from build123d import *

# Parameters (mm, degrees)
SKETCH1_W                    = 406.4
SKETCH1_H                    = 44.196
BASE_FLANGE1_DEPTH           = 1.88
EDGE_FLANGE1_STRIP_W         = 8.9932
EDGE_FLANGE1_STRIP_H         = 1.88
EDGE_FLANGE1_STRIP_CUT_DEPTH = 44.196
EDGE_FLANGE1_DEPTH           = 44.196
CUT_EXTRUDE1_REACH           = 411.347
FILLET1_R                    = 5


# Sheet-metal steps are written as plain solids
with BuildPart() as part:
    # Sketch1 → Base-Flange1 (new body)
    with BuildSketch(Plane.XY):
        with Locations((203.2, 22.098)):
            Rectangle(SKETCH1_W, SKETCH1_H)
        with BuildLine():
            Line((139.7, 36.2225), (400.05, 36.2225))
            ThreePointArc((400.05, 36.2225), (402.2725, 34), (400.05, 31.7775))
            Line((400.05, 31.7775), (139.7, 31.7775))
            ThreePointArc((139.7, 31.7775), (137.4775, 34), (139.7, 36.2225))
        make_face(mode=Mode.SUBTRACT)
        with BuildLine():
            Line((139.7, 12.2225), (400.05, 12.2225))
            ThreePointArc((400.05, 12.2225), (402.2725, 10), (400.05, 7.7775))
            Line((400.05, 7.7775), (139.7, 7.7775))
            ThreePointArc((139.7, 7.7775), (137.4775, 10), (139.7, 12.2225))
        make_face(mode=Mode.SUBTRACT)
    extrude(amount=-BASE_FLANGE1_DEPTH)

    # Edge-Flange1 strip (across the edge) → Edge-Flange1 strip cut (cut)
    with BuildSketch(Plane.XZ.offset(-44.196)):
        with Locations((-1.88, -0.94)):
            Rectangle(EDGE_FLANGE1_STRIP_W, EDGE_FLANGE1_STRIP_H)
    extrude(amount=EDGE_FLANGE1_STRIP_CUT_DEPTH, mode=Mode.SUBTRACT)

    # Edge-Flange1 section (across the edge) → Edge-Flange1 (add)
    with BuildSketch(Plane.XZ.offset(-44.196)):
        with BuildLine():
            Line((0, 0.7366), (0, 21.234))
            Line((0, 21.234), (1.88, 21.234))
            Line((1.88, 21.234), (1.88, 0.7366))
            ThreePointArc((1.88, 0.7366), (2.095745145, 0.215745145), (2.6166, 0))
            Line((2.6166, 0), (2.6166, -1.88))
            ThreePointArc((2.6166, -1.88), (0.766384396, -1.113615604), (0, 0.7366))
        make_face()
    extrude(amount=EDGE_FLANGE1_DEPTH)

    # Sketch9 → Cut-Extrude1 (cut, up to next)
    with BuildSketch(Plane.ZY, mode=Mode.PRIVATE) as cut_extrude1_sk1:
        with BuildLine():
            Line((11.145, 41.656), (14.305, 41.656))
            ThreePointArc((14.305, 41.656), (17.805, 38.156), (14.305, 34.656))
            Line((14.305, 34.656), (11.145, 34.656))
            ThreePointArc((11.145, 34.656), (7.645, 38.156), (11.145, 41.656))
        make_face()
    cut_extrude1_tool1 = extrude(cut_extrude1_sk1.sketch, amount=-CUT_EXTRUDE1_REACH, mode=Mode.PRIVATE) & part.part
    # Sketch9 → Cut-Extrude1 (cut, up to next)
    with BuildSketch(Plane.ZY, mode=Mode.PRIVATE) as cut_extrude1_sk2:
        with BuildLine():
            Line((11.145, 9.54), (14.305, 9.54))
            ThreePointArc((14.305, 9.54), (17.805, 6.04), (14.305, 2.54))
            Line((14.305, 2.54), (11.145, 2.54))
            ThreePointArc((11.145, 2.54), (7.645, 6.04), (11.145, 9.54))
        make_face()
    cut_extrude1_tool2 = extrude(cut_extrude1_sk2.sketch, amount=-CUT_EXTRUDE1_REACH, mode=Mode.PRIVATE) & part.part
    add(cut_extrude1_tool1.solids().sort_by_distance((0, 38.156, 12.725))[0], mode=Mode.SUBTRACT)
    add(cut_extrude1_tool2.solids().sort_by_distance((0, 6.04, 12.725))[0], mode=Mode.SUBTRACT)

    # Fillet1
    fillet1_edges = [part.edges().sort_by_distance(p)[0] for p in [
        (0.94, 44.196, 21.234),
        (0.94, 0, 21.234),
        (406.4, 44.196, -0.94),
        (406.4, 0, -0.94),
    ]]
    fillet(fillet1_edges, radius=FILLET1_R)


solid = part.part
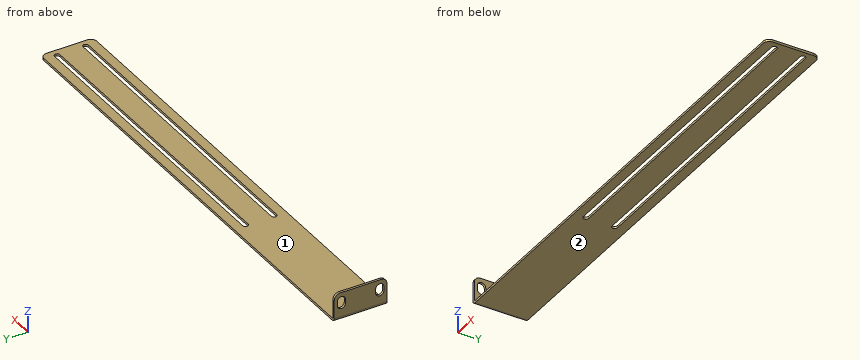
Geometry check sheet. Reference: the model listing, model coordinates, mm. Face numbers are marked on the shaded views. A direction names the side the tool comes from. Give positions to 0.01 mm unless a question says otherwise; leave off trailing zeros. Loops run counter-clockwise (first coordinate to the right, second up) from the corner with the lowest first, then second, coordinate; pieces in that order, holes last.
(1) Thickness scan on L1, parallel to Z at x = 121, y = 41.5; L2, parallel to X at y = 23, z = 10; L3, parallel to X at y = 28, z = -0.5. Record the ranges inside material, lowest first.
From the geometry:
L1: z = -1.88 to 0
L2: x = 0 to 1.88
L3: x = 0.31 to 406.4
(2) Section check C-C on x = 124. Record the cut outline in (y, z), then the cut area to 3 significant figures.
From the geometry:
outline: (0, -1.88) - (44.2, -1.88) - (44.2, 0) - (0, 0) - close
area: 83.1 mm2
(3) Set-up check for the marked faces 1 and 2: record each of +Z, -Z, +X, -X, +Y, -Y from which the full face is reachable in a straight line by a thin tool's end or side.
From the geometry:
face 1: +Z, +X, +Y, -Y
face 2: -Z, +X, -X, +Y, -Y
(4) Section check A-A on x = 281.5. Record the cut outline in (y, z).
From the geometry:
outline: (0, -1.88) - (7.78, -1.88) - (7.78, 0) - (0, 0) - close; (12.22, -1.88) - (31.78, -1.88) - (31.78, 0) - (12.22, 0) - close; (36.22, -1.88) - (44.2, -1.88) - (44.2, 0) - (36.22, 0) - close
(5) Depth check by flat-ended pin: pin 1 Ø1.5 at (y, z) = (11, 10) entering from -X; pin 2 Ø1 at (x, y) = (354.5, 30.5) entering from +Z. Enter the tip coordinate at first touch or a pass-through.
From the geometry:
pin 1: stops at x = 0
pin 2: stops at z = 0
(6) Section check B-B on y = 23. Record the cut outline in (x, z), then the cut area to 3 significant figures.
From the geometry:
outline: (0, 0.74) arc R2.62 ccw to (2.62, -1.88) - (406.4, -1.88) - (406.4, 0) - (2.62, 0) arc R0.74 cw to (1.88, 0.74) - (1.88, 21.23) - (0, 21.23) - close
area: 803 mm2
